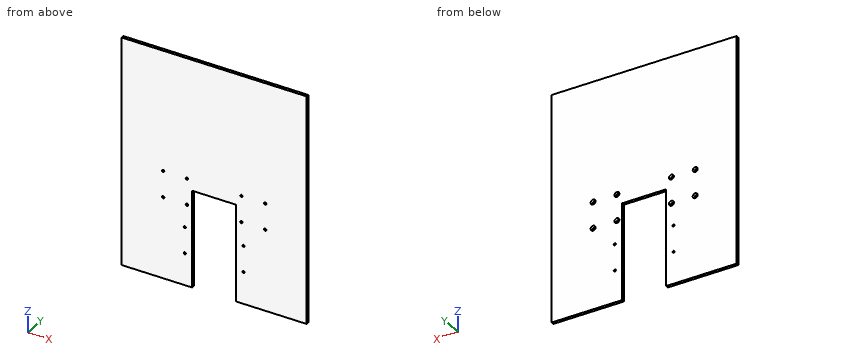
from build123d import *

# Parameters (mm, degrees)
SKETCH1_W                                       = 350
SKETCH1_H                                       = 250
BOSS_EXTRUDE1_DEPTH                             = 5.3
SKETCH4_W                                       = 133.5
SKETCH4_H                                       = 5.3
BOSS_EXTRUDE3_DEPTH                             = 185
F_4_0MM_DOWEL_HOLE1_D                           = 4
CSK_FOR_M4_FLAT_HEAD_MACHINE_SCREW2_D           = 4.5
CSK_FOR_M4_FLAT_HEAD_MACHINE_SCREW2_CSINK_D     = 9.4
CSK_FOR_M4_FLAT_HEAD_MACHINE_SCREW2_CSINK_ANGLE = 90


with BuildPart() as part:
    # Sketch1 → Boss-Extrude1 (new body)
    with BuildSketch(Plane(origin=(0, 0, 0), x_dir=(1, 0, 0), z_dir=(0, 1, 0))):
        with Locations((-85.330578512, -202.479338843)):
            Rectangle(SKETCH1_W, SKETCH1_H)
    extrude(amount=BOSS_EXTRUDE1_DEPTH)

    # Sketch4 → Boss-Extrude3 (add)
    with BuildSketch(Plane(origin=(0, 0, 77.479338843), x_dir=(-1, 0, 0), z_dir=(0, 0, -1))):
        with Locations((193.580578512, 2.65)):
            Rectangle(SKETCH4_W, SKETCH4_H)
        with Locations((-22.919421488, 2.65)):
            Rectangle(SKETCH4_W, SKETCH4_H)
    extrude(amount=BOSS_EXTRUDE3_DEPTH)

    # Ø4.0mm Dowel Hole1 (through all)
    with Locations(Plane(origin=(0, 5.3, 0), x_dir=(1, 0, 0), z_dir=(0, 1, 0))):
        with Locations((-181.830578512, -47.479338843), (-181.830578512, -97.479338843), (-136.830578512, -97.479338843), (-136.830578512, -47.479338843), (-33.830578512, -47.479338843), (11.169421488, -47.479338843), (11.169421488, -97.479338843), (-33.830578512, -97.479338843), (-29.830578512, -3.479338843), (-29.830578512, 46.520661157), (-140.830578512, 46.520661157), (-140.830578512, -3.479338843)):
            Hole(F_4_0MM_DOWEL_HOLE1_D / 2)

    # CSK for M4 Flat Head Machine Screw2 (through all)
    with Locations(Plane(origin=(0, 5.3, 0), x_dir=(1, 0, 0), z_dir=(0, 1, 0))):
        with Locations((-181.830578512, -47.479338843), (-136.830578512, -47.479338843), (-181.830578512, -97.479338843), (-136.830578512, -97.479338843), (-33.830578512, -47.479338843), (11.169421488, -47.479338843), (11.169421488, -97.479338843), (-33.830578512, -97.479338843)):
            CounterSinkHole(CSK_FOR_M4_FLAT_HEAD_MACHINE_SCREW2_D / 2, CSK_FOR_M4_FLAT_HEAD_MACHINE_SCREW2_CSINK_D / 2, counter_sink_angle=CSK_FOR_M4_FLAT_HEAD_MACHINE_SCREW2_CSINK_ANGLE)


solid = part.part
The listing builds one solid part. Answer for the finished solid, in the listing's coordinates (mm). Round coordinates to 2 decimals unless told otherwise and drop trailing zeros. Order: outer loops, then holes, each group sorted by start corner. A loop starts at its lowest first (then second) coordinate and runs counter-clockwise, first axis right, second up. Notation, with made-up numbers: (25.25, -30.5) -> (51.25, -30.5) arc R25 cw to (51.25, -6.5) -> close; hole circle Ø8 at (78, 66.5). An arc over 180 degrees is marked (long way). Write each question's results on one line, items separated by ' | '. Start each with the question number.
Q1. Straight lines are drawn through the part: probe 1 along X at (y, z) = (0.35, -13); probe 2 along Z at (x, y) = (-89.5, 1.6); probe 3 along X at (y, z) = (3.8, -45). For each, find the intervals that lie inside material, in ascending order. Write a range as from..to.
Q2. Find section B-B (y = 1.95). Give the number of separate pieces and of enclosed holes in the cut face, then the cut area to 3 significant figures.
Q3. Find section C-C (x = -102.5). Determine the outline of the cut face in (y, z), then the cut area to 4 significant figures.
Q4. Each of these flat-tipped pins is pushed along its axis until it touches: pin 1 (3 mm diameter, centred on x = -140.83, z = 3.48, fed in from +Y); pin 2 (7 mm diameter, centred on x = 11.17, z = 97.48, fed in from +Y); pin 3 (5 mm diameter, centred on x = -136.83, z = 47.48, fed in from +Y); pin 4 (1.6 mm diameter, centred on x = -70, y = 2.5, fed in from -Z). Where does it stop, or does it pass through?
Q5. Find section A-A (z = -60). Determine the outline of the cut face in (x, y), then the cut area to 3 significant figures.
Worked answers:
1) probe 1: x = -260.33..-126.83, -43.83..89.67 | probe 2: z = 77.48..327.48 | probe 3: x = -260.33..-142.13, -139.53..-126.83, -43.83..-31.13, -28.53..89.67
2) separate pieces: 1 | enclosed holes: 12 | area: 137,000 mm2
3) outline: (0, 77.48) -> (5.3, 77.48) -> (5.3, 327.48) -> (0, 327.48) -> close | area: 1,325 mm2
4) pin 1: passes through | pin 2: stops at y = 4.1 | pin 3: stops at y = 3.1 | pin 4: stops at z = 77.48
5) outline: (-260.33, 0) -> (-126.83, 0) -> (-126.83, 5.3) -> (-260.33, 5.3) -> close; (-43.83, 0) -> (89.67, 0) -> (89.67, 5.3) -> (-43.83, 5.3) -> close | area: 1,420 mm2
